Could you check a few things on this model? Use its own coordinates, in mm. A direction names the side the tool comes from. Give positions to 0.01 mm unless a question says otherwise; leave off trailing zeros. Order: outer loops, then holes, each group sorted by start corner. A loop starts at its lowest first (then second) coordinate and runs counter-clockwise, first axis right, second up. Notation, with made-up numbers: M -12.5,-25 L 31.5,-25 A26 ccw 31.5,9 Z; hole C 32,61 d8. An arc over 180 degrees is marked long. Return JSON: item names as keys, results as strings. Group by question number.
```python
from build123d import *

# Parameters (mm, degrees)
CUT_EXTRUDE1_START = 2.2987
CUT_EXTRUDE1_DEPTH = 10.922
CIRPATTERN1_COUNT  = 18
SKETCH4_R          = 2.0828
CUT_EXTRUDE2_DEPTH = 27.762350537
CUT_EXTRUDE3_DEPTH = 1.5621
CIRPATTERN2_COUNT  = 2
CIRPATTERN2_ANGLE  = 90


with BuildPart() as part:
    # Sketch2 → Revolve1 (revolve)
    with BuildSketch(Plane(origin=(0, 0, 0), x_dir=(0, 0, -1), z_dir=(1, 0, 0)), mode=Mode.PRIVATE) as revolve1_sk:
        with BuildLine():
            Line((-10.3124, 6.35), (10.3124, 6.35))
            Line((10.3124, 6.35), (10.3124, 17.4625))
            Line((10.3124, 17.4625), (9.46785, 17.4625))
            ThreePointArc((9.46785, 17.4625), (8.847668679, 16.777633999), (8.6233, 15.88135))
            Line((8.6233, 15.88135), (8.6233, 14.3002))
            Line((8.6233, 14.3002), (-2.2987, 14.3002))
            Line((-2.2987, 14.3002), (-2.2987, 15.88135))
            ThreePointArc((-2.2987, 15.88135), (-2.523068679, 16.777633999), (-3.14325, 17.4625))
            Line((-3.14325, 17.4625), (-3.9878, 17.4625))
            Line((-3.9878, 17.4625), (-3.9878, 10.3124))
            Line((-3.9878, 10.3124), (-10.3124, 10.3124))
            Line((-10.3124, 10.3124), (-10.3124, 6.35))
        make_face()
    revolve(revolve1_sk.sketch.rotate(Axis((0, 0, 10.3124), (0, 0, -1)), 90), axis=Axis((0, 0, 10.3124), (0, 0, -1)))

    # Sketch3 → Cut-Extrude1 (cut)
    with BuildSketch(Plane.XY.offset(CUT_EXTRUDE1_START)):
        with BuildLine():
            Line((-0.635, 12.842092967), (0.635, 12.842092967))
            Line((0.635, 12.842092967), (1.287830721, 14.242092967))
            ThreePointArc((1.287830721, 14.242092967), (0, 14.3002), (-1.287830721, 14.242092967))
            Line((-1.287830721, 14.242092967), (-0.635, 12.842092967))
        make_face()
    cut_extrude1 = extrude(amount=-CUT_EXTRUDE1_DEPTH, mode=Mode.SUBTRACT)

    # CirPattern1: Cut-Extrude1 ×18 about axis
    cirpattern1_axis = Axis((0, 0, 0), (0, 0, 1))
    for i in range(1, CIRPATTERN1_COUNT):
        add(cut_extrude1.rotate(cirpattern1_axis, i * 360 / CIRPATTERN1_COUNT), mode=Mode.SUBTRACT)

    # Sketch4 → Cut-Extrude2 (cut, through all)
    with BuildSketch(Plane(origin=(0, 0, 0), x_dir=(1, 0, 0), z_dir=(0, 1, 0))):
        with Locations(Location((0, -7.1501, 0), (0, 0, 90))):
            Circle(SKETCH4_R)
    cut_extrude2 = extrude(amount=CUT_EXTRUDE2_DEPTH, mode=Mode.SUBTRACT)

    # Sketch5 → Revolve2 (revolve)
    with BuildSketch(Plane.XY.offset(7.1501), mode=Mode.PRIVATE) as revolve2_sk:
        Polygon((1.5748, 10.099878114), (2.0828, 9.591878114), (2.0828, 6.985), (1.4478, 6.35), (0, 6.35), (0, 10.099878114), align=None)
    revolve2 = revolve(revolve2_sk.sketch.rotate(Axis((0, 0, 7.1501), (0, 1, 0)), 90), axis=Axis((0, 0, 7.1501), (0, 1, 0)))

    # Sketch6 → Cut-Extrude3 (cut)
    with BuildSketch(Plane(origin=(0, 10.099878114, 0), x_dir=(1, 0, 0), z_dir=(0, 1, 0))):
        Polygon((0, -5.947594859), (-1.0414, -6.54884743), (-1.0414, -7.75135257), (0, -8.352605141), (1.0414, -7.75135257), (1.0414, -6.54884743), align=None)
    cut_extrude3 = extrude(amount=-CUT_EXTRUDE3_DEPTH, mode=Mode.SUBTRACT)

    # CirPattern2: Cut-Extrude2, Revolve2, Cut-Extrude3 ×2 about axis
    cirpattern2_axis = Axis((0, 0, 0), (0, 0, -1))
    add([cut_extrude2.rotate(cirpattern2_axis, i * CIRPATTERN2_ANGLE / (CIRPATTERN2_COUNT - 1)) for i in range(1, CIRPATTERN2_COUNT)], mode=Mode.SUBTRACT)
    add([revolve2.rotate(cirpattern2_axis, i * CIRPATTERN2_ANGLE / (CIRPATTERN2_COUNT - 1)) for i in range(1, CIRPATTERN2_COUNT)])
    add([cut_extrude3.rotate(cirpattern2_axis, i * CIRPATTERN2_ANGLE / (CIRPATTERN2_COUNT - 1)) for i in range(1, CIRPATTERN2_COUNT)], mode=Mode.SUBTRACT)


solid = part.part
```
1. I need wall thicknesses on L1, parallel to X at y = -10, z = -5.5; L2, parallel to Z at x = 0, y = 9; L3, parallel to X at y = 12.5, z = 1. Which ranges of each line are inside material? Lowest first, please. Write a range as from..to.
2. Which directions (+Z, -Z, +X, -X, +Y, -Y) give clear straight access to the entire face, cutting with the end or side of a thin tool? Please do faces 1 (the flat face through (3.73, -13.04, -3.09)), 2 (the flat face through (7.965, -10.981, -3.086)), 3 (the flat face through (-0.51, 9.33, 6.24)), 4 (the cylindrical face through (-13.44, 4.88, -3.09)).
3. Imagine slicing it at A-A, the plane z = 4.5. Please give me the cut outline in (x, y), plus the area to 3 significant figures.
4. For pin 1 (3 mm diameter, centred on y = -5.5, z = -1, fed in from -X); pin 2 (1.3 mm diameter, centred on x = 9, z = 7, fed in from +Y); pin 3 (1.7 mm diameter, centred on x = 0, z = 7.5, fed in from +Y), each with a flat end and sliding along its axis, tell me the tip position at first contact or that it passes through.
5. If we mould it in two halves opening along Z, with no side actions, what happens to faces 5 (the flat face through (7, 0, 10.312)), 6 (the flat face through (12.65, -2.22, -3.09))? For each: pulls with the +Z half, pulls with the -Z half, needs draft (parallel to the pull), parting line crosses it, or undercut.
Values:
{
 "1": {"L1": "x = -10.22..-9.96, -8.06..8.06, 9.96..10.22", "L2": "z = -10.31..5.95, 8.35..10.31", "L3": "x = -6.95..-5.64, -3.78..3.78, 5.64..6.95"},
 "2": {"face 1": "-Y", "face 2": "+X", "face 3": "+Y", "face 4": "-X, +Y"},
 "3": {"outline": "C 0,0 d20.62; hole C 0,0 d12.7", "area": "207 mm²"},
 "4": {"pin 1": "stops at x = -13.73", "pin 2": "stops at y = 6.05", "pin 3": "stops at y = 10.1"},
 "5": {"face 5": "pulls with the +Z half", "face 6": "undercut"}
}
